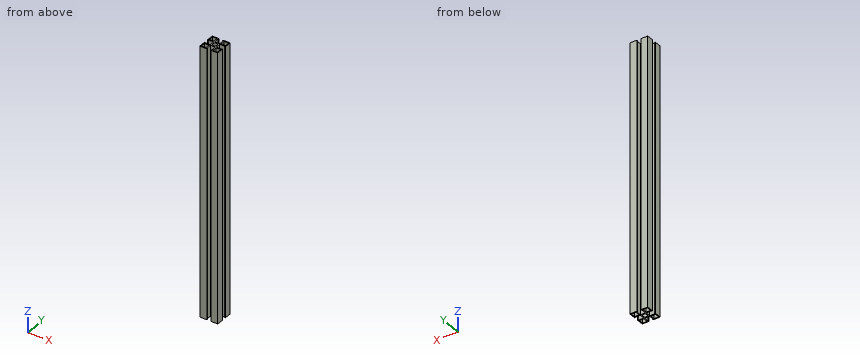
from build123d import *

# Parameters (mm, degrees)
SKETCH_1_R      = 4.5
SKETCH_1_W      = 10
SKETCH_1_H      = 10
EXTRUDE_1_DEPTH = 600


with BuildPart() as part:
    # 草图1 → 凸台-拉伸1 (new body)
    with BuildSketch(Plane.XY):
        Polygon((0, 0), (15.5, 0), (15.5, 1.949576264), (14.5, 1.949576264), (14.5, 13.449576264), (25.5, 13.449576264), (25.5, 1.949576264), (24.5, 1.949576264), (24.5, 0), (40, 0), (40, 15.5), (38.050423736, 15.5), (38.050423736, 14.5), (26.550423736, 14.5), (26.550423736, 25.5), (38.050423736, 25.5), (38.050423736, 24.5), (40, 24.5), (40, 40), (24.5, 40), (24.5, 38.050423736), (25.5, 38.050423736), (25.5, 26.550423736), (14.5, 26.550423736), (14.5, 38.050423736), (15.5, 38.050423736), (15.5, 40), (0, 40), (0, 24.5), (1.949576264, 24.5), (1.949576264, 25.5), (13.449576264, 25.5), (13.449576264, 14.5), (1.949576264, 14.5), (1.949576264, 15.5), (0, 15.5), align=None)
        with Locations((20, 20)):
            Circle(SKETCH_1_R, mode=Mode.SUBTRACT)
        with Locations((7, 33)):
            Rectangle(SKETCH_1_W, SKETCH_1_H, mode=Mode.SUBTRACT)
        with Locations((7, 7)):
            Rectangle(SKETCH_1_W, SKETCH_1_H, mode=Mode.SUBTRACT)
        with Locations((33, 33)):
            Rectangle(SKETCH_1_W, SKETCH_1_H, mode=Mode.SUBTRACT)
        with Locations((33, 7)):
            Rectangle(SKETCH_1_W, SKETCH_1_H, mode=Mode.SUBTRACT)
    extrude(amount=EXTRUDE_1_DEPTH)


solid = part.part
Design review of the part built by this model. Coordinates are the model's own, in mm. Coordinates: 2 decimals unless noted, no trailing zeros. One line per item, written item: value.
1) We need section A-A, the plane z = 416. Count the separate pieces of the cut face and the enclosed holes in it, then the cut area to 3 significant figures.
Output values:
separate pieces: 1
enclosed holes: 5
area: 560 mm2
2) To check wall thickness, follow probe 1 along Y at (x, z) = (11.5, 190); probe 2 along Y at (x, z) = (19.5, 493). State the ranges of each line that lie inside material, in increasing order. Write a range as [from, to].
Output values:
probe 1: y = [0, 2], [12, 14.5], [25.5, 28], [38, 40]
probe 2: y = [13.45, 15.53], [24.47, 26.55]
3) Clearance check with flat-ended pins moving along their axes: P1, Ø4, axis at y = 21, z = 351, coming from the -X side; P2, Ø3.5, axis at y = 18, z = 357.5, coming from the +X side. State where each tip first meets the part, or that it passes through.
Output values:
P1: stops at x = 13.45
P2: stops at x = 26.55
